Study the drawing (mm; zero at the part's minimum x, y, z) and answer. Give positions to 0.01 mm unless a question says otherwise; leave off trailing zeros. Order: outer loops, then holes, each group sorted by start corner. A loop starts at its lowest first (then second) coordinate and runs counter-clockwise, first axis right, second up. Notation, with made-up numbers: (12, 13) - (28, 13) arc R15 cw to (28, 39) - close; hole circle Ø1 at (12.5, -12.75). An arc over 180 degrees is marked (long way). Write each question's results on one line, items separated by ' | '. Start each with the question number.
Q1. Flat-ended cylindrical pins translate along their axes: P1, Ø3, axis at x = 25, z = 19.5, coming from the -Y side; P2, Ø3, axis at y = 7, z = 8, coming from the -X side; P3, Ø5, axis at y = 11, z = 7.5, coming from the -X side. Find the tip coordinate at first contact, or state that the pin passes through.
Q2. For a pull along Y with two mould halves and no side action, classify the marked faces 1, 2 and 3 as +Y half, -Y half, draft (parallel to the pull), parting line (faces both ways), or undercut.
Q3. Find section C-C on z = 3.75. Give the vertices of the cut face in (x, y).
Q4. Find the intervals of material crossed by line 1 along Y through (x, z) = (21, 13.75); line 2 along Y through (x, z) = (25.5, 18); line 3 along Y through (x, z) = (22.5, 3), in increasing order. Write a range as from..to.
Q5. Find section A-A on y = 21. Give the vertices of the cut face in (x, z), and give its area (3 significant figures).
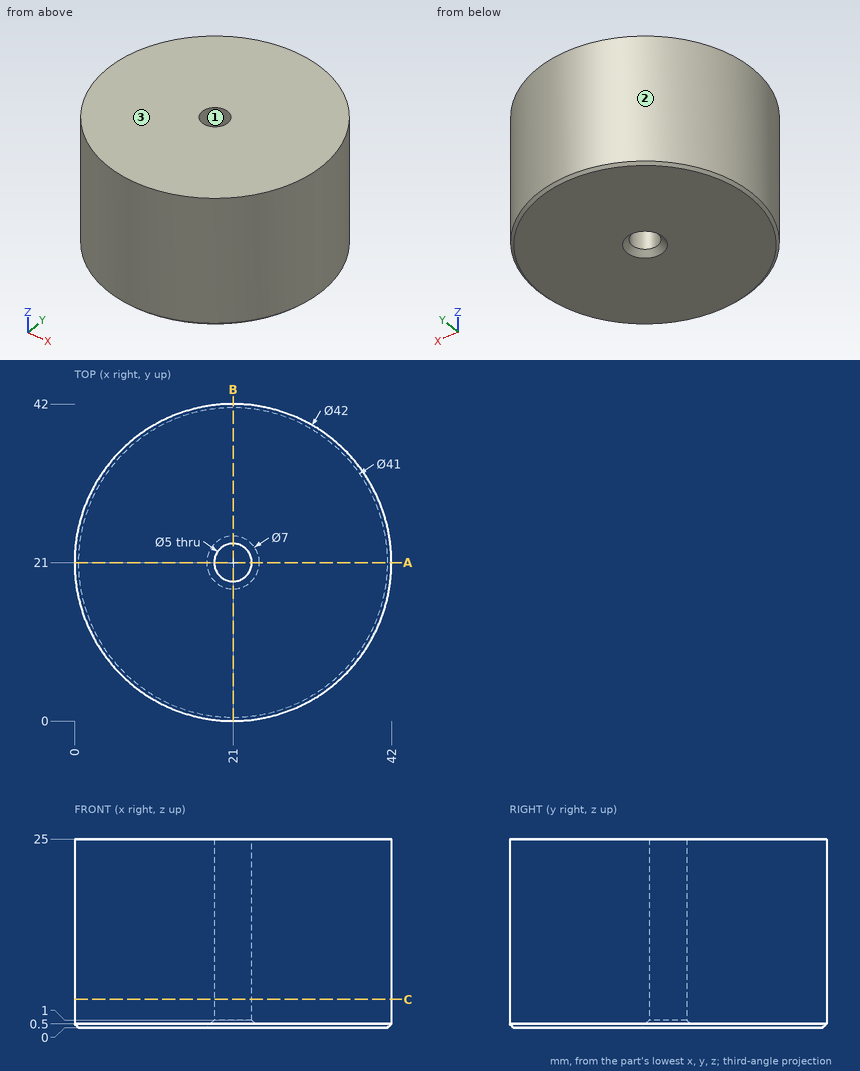
Working result:
1) P1: y = 0.15 | P2: x = 4.13 | P3: x = 1.38
2) face 1: undercut | face 2: parting line | face 3: draft
3) outline: circle Ø42 at (21, 21); hole circle Ø5 at (21, 21)
4) line 1: 0..18.5, 23.5..42 | line 2: 0.49..41.51 | line 3: 0.05..19, 23..41.95
5) outline: (0, 0.5) - (0.5, 0) - (17.5, 0) - (18.5, 1) - (18.5, 25) - (0, 25) - close; (23.5, 1) - (24.5, 0) - (41.5, 0) - (42, 0.5) - (42, 25) - (23.5, 25) - close | area: 924 mm²
